Source: CAD feature listing. Evaluate the final solid. Frame: model axes, mm. A direction names the side the tool comes from. Round coordinates to 2 decimals unless told otherwise and drop trailing zeros. Order: outer loops, then holes, each group sorted by start corner. A loop starts at its lowest first (then second) coordinate and runs counter-clockwise, first axis right, second up. Notation, with made-up numbers: (22.5, 86.25) - (64.5, 86.25) arc R36 ccw to (64.5, 120.25) - close; hole circle Ø7 at (-31.75, 73.5). An arc over 180 degrees is marked (long way). Use one line per item in the form item = value. Start each with the question number.
Q1. Ray query, line 1 (X direction, y = 0.5, z = 4.4); line 2 (Y direction, x = 1.5, z = 3.35); line 3 (X direction, y = -2.75, z = 3.8). Return the intervals inside material, ascending. Write a range as [from, to].
Q2. Cut plane C-C, the plane z = 2.85. Give the number of separate pieces and of enclosed holes in the cut face, and give its area (3 significant figures).
Q3. Cut plane A-A, the plane x = -10. Return the cut outline in (y, z), and give its area (3 significant figures).
Q4. Cut plane B-B, the plane y = 0. Return the cut outline in (x, z), and give its area (3 significant figures).
Q5. Draft query along Y for faces 1 (the cylindrical face through (1.576, -5.824, 1.535)), 2 (the cylindrical face through (-14.735, 8.091, 2.958)), 3 (the cylindrical face through (1.576, -5.081, 3.595)), 4 (the flat face through (-5, 3, 0)). Return one class per face: released by +Y, released by -Y, zero draft, split by the parting line, or undercut.
Q6. Set-up query: faces 5 (the flat face through (-5.433, 9, 3)), 6 (the flat face through (-5.704, -3.6, 3)), 7 (the flat face through (-12.199, -3.6, 3)), 8 (the flat face through (-6, 9, 1)). Return all of +Z, -Z, +X, -X, +Y, -Y with unobstructed straight access to the full face (end or side cutting, diameter ignored); none if empty.
Q7. Pin query (flat end, axial travel): pin 1 Ø3 at (x, y) = (-5, 10.5) entering from +Z; pin 2 Ø3 at (y, z) = (-3.5, 3) entering from +X; pin 3 Ø3 at (x, z) = (-11, 3.5) entering from +Y. Return the tip coordinate at first contact, or that it passes through.
Q8. Cut plane D-D, the plane x = 3. Return the cut outline in (y, z).
from build123d import *

# Parameters (mm, degrees)
BOSS_EXTRUDE1_DEPTH            = 4
BOSS_EXTRUDE2_DEPTH            = 1
CUT_EXTRUDE1_DEPTH             = 1
SKETCH4_W                      = 8.3
SKETCH4_H                      = 5
BOSS_EXTRUDE3_DEPTH            = 10
SKETCH5_W                      = 4
SKETCH5_H                      = 0.3
BOSS_EXTRUDE4_DEPTH            = 17.182840277
SKETCH6_W                      = 5
SKETCH6_H                      = 10
BOSS_EXTRUDE5_DEPTH            = 9
SKETCH7_W                      = 5
SKETCH7_H                      = 11
BOSS_EXTRUDE6_DEPTH            = 2.7
BOSS_EXTRUDE7_DEPTH            = 1
SKETCH9_W                      = 2
SKETCH9_H                      = 4
BOSS_EXTRUDE8_DEPTH            = 1.58656304
SKETCH10_W                     = 0.5
SKETCH10_H                     = 3.5
BOSS_EXTRUDE9_DEPTH            = 3.5
SKETCH11_W                     = 0.5
SKETCH11_H                     = 3.5
BOSS_EXTRUDE10_DEPTH           = 3.5
SKETCH12_W                     = 0.5
SKETCH12_H                     = 3.5
BOSS_EXTRUDE11_DEPTH           = 3.5
F_2_5_2_5_DIAMETER_HOLE1_D     = 2.5
F_2_5_2_5_DIAMETER_HOLE1_DEPTH = 6
F_1_5_1_5_DIAMETER_HOLE1_D     = 1.5
F_1_5_1_5_DIAMETER_HOLE1_DEPTH = 3.337462294
F_1_5_1_5_DIAMETER_HOLE2_D     = 1.5
F_1_5_1_5_DIAMETER_HOLE2_DEPTH = 3.641193774
F_1_5_1_5_DIAMETER_HOLE3_D     = 1.5
F_1_5_1_5_DIAMETER_HOLE3_DEPTH = 10.667359759
FILLET1_R                      = 0.5
FILLET2_R                      = 1


with BuildPart() as part:
    # Sketch1 → Boss-Extrude1 (new body)
    with BuildSketch(Plane(origin=(0, 0, 1), x_dir=(-1, 0, 0), z_dir=(0, 0, -1))):
        with BuildLine():
            Line((4.743251359, 8.08281548), (4.036144578, 7.375708699))
            Line((4.036144578, 7.375708699), (12.336144578, 7.375708699))
            Line((12.336144578, 7.375708699), (12.336144578, 9.634817645))
            Line((12.336144578, 9.634817645), (12.079792775, 9.67251644))
            Line((12.079792775, 9.67251644), (12.036144578, 9.375708699))
            Line((12.036144578, 9.375708699), (12.036144578, 8.375708699))
            Line((12.036144578, 8.375708699), (5.450358141, 8.375708699))
            ThreePointArc((5.450358141, 8.375708699), (5.067674708, 8.299588231), (4.743251359, 8.08281548))
        make_face()
    extrude(amount=-BOSS_EXTRUDE1_DEPTH)

    # Sketch2 → Boss-Extrude2 (add)
    with BuildSketch(Plane.XY.offset(5)):
        with BuildLine():
            Line((-12.336144578, 7.375708699), (-12.336144578, 9.634817645))
            Line((-12.336144578, 9.634817645), (-12.079792775, 9.67251644))
            Line((-12.079792775, 9.67251644), (-12.036144578, 9.375708699))
            Line((-12.036144578, 9.375708699), (-12.036144578, 8.375708699))
            Line((-12.036144578, 8.375708699), (-5.450358141, 8.375708699))
            ThreePointArc((-5.450358141, 8.375708699), (-5.067674708, 8.299588231), (-4.743251359, 8.08281548))
            Line((-4.743251359, 8.08281548), (-4.036144578, 7.375708699))
            Line((-4.036144578, 7.375708699), (-12.336144578, 7.375708699))
        make_face()
    extrude(amount=BOSS_EXTRUDE2_DEPTH)

    # Sketch3 → Cut-Extrude1 (cut)
    with BuildSketch(Plane.XY.offset(6)):
        Polygon((-12.036144578, 8.375708699), (-12.036144578, 9.375708699), (-12.079792775, 9.67251644), (-12.336144578, 9.634817645), (-12.336144578, 8.375708699), align=None)
    extrude(amount=-CUT_EXTRUDE1_DEPTH, mode=Mode.SUBTRACT)

    # Sketch4 → Boss-Extrude3 (add)
    with BuildSketch(Plane.XZ.offset(-7.375708699)):
        with Locations((-8.186144578, 3.5)):
            Rectangle(SKETCH4_W, SKETCH4_H)
    extrude(amount=BOSS_EXTRUDE3_DEPTH)

    # Sketch5 → Boss-Extrude4 (add)
    with BuildSketch(Plane(origin=(-10.431763466, -1.534082863, 0), x_dir=(0, 0, -1), z_dir=(0.989359135, 0.14549399, 0))):
        with Locations((-3, 11.177129757)):
            Rectangle(SKETCH5_W, SKETCH5_H)
    extrude(amount=BOSS_EXTRUDE4_DEPTH)

    # Sketch6 → Boss-Extrude5 (add)
    with BuildSketch(Plane(origin=(-4.036144578, 0, 0), x_dir=(0, 0, -1), z_dir=(1, 0, 0))):
        with Locations((-3.5, 2.375708699)):
            Rectangle(SKETCH6_W, SKETCH6_H)
    extrude(amount=BOSS_EXTRUDE5_DEPTH)

    # Sketch7 → Boss-Extrude6 (add)
    with BuildSketch(Plane.ZY.offset(12.336144578)):
        with Locations((3.5, 2.875708699)):
            Rectangle(SKETCH7_W, SKETCH7_H)
    extrude(amount=BOSS_EXTRUDE6_DEPTH)

    # Sketch8 → Boss-Extrude7 (add)
    with BuildSketch(Plane(origin=(0, 0, 1), x_dir=(-1, 0, 0), z_dir=(0, 0, -1))):
        with BuildLine():
            Line((15.036144578, 8.375708699), (15.036144578, -2.624291301))
            Line((15.036144578, -2.624291301), (-4.963855422, -2.624291301))
            Line((-4.963855422, -2.624291301), (-4.963855422, 7.375708699))
            Line((-4.963855422, 7.375708699), (4.036144578, 7.375708699))
            Line((4.036144578, 7.375708699), (4.743251359, 8.08281548))
            ThreePointArc((4.743251359, 8.08281548), (5.067674708, 8.299588231), (5.450358141, 8.375708699))
            Line((5.450358141, 8.375708699), (15.036144578, 8.375708699))
        make_face()
    extrude(amount=BOSS_EXTRUDE7_DEPTH)

    # Sketch9 → Boss-Extrude8 (add)
    with BuildSketch(Plane(origin=(0, 8.375708699, 0), x_dir=(-1, 0, 0), z_dir=(0, 1, 0))):
        with Locations((6.43261709, 3)):
            Rectangle(SKETCH9_W, SKETCH9_H)
    extrude(amount=BOSS_EXTRUDE8_DEPTH)

    # Sketch10 → Boss-Extrude9 (add)
    with BuildSketch(Plane.XZ.offset(2.624291301)):
        with Locations((-5.453504337, 3)):
            Rectangle(SKETCH10_W, SKETCH10_H)
    extrude(amount=BOSS_EXTRUDE9_DEPTH)

    # Sketch11 → Boss-Extrude10 (add)
    with BuildSketch(Plane.XZ.offset(2.624291301)):
        with Locations((1.572661648, 3)):
            Rectangle(SKETCH11_W, SKETCH11_H)
    extrude(amount=BOSS_EXTRUDE10_DEPTH)

    # Sketch12 → Boss-Extrude11 (add)
    with BuildSketch(Plane.XZ.offset(2.624291301)):
        with Locations((-11.948682285, 3)):
            Rectangle(SKETCH12_W, SKETCH12_H)
    extrude(amount=BOSS_EXTRUDE11_DEPTH)

    # Ø2.5 (2.5) Diameter Hole1
    with Locations(Plane.XY.offset(6)):
        with Locations((-9.786144578, 0.375708699), (-0.286144578, 0.375708699)):
            Hole(F_2_5_2_5_DIAMETER_HOLE1_D / 2, depth=F_2_5_2_5_DIAMETER_HOLE1_DEPTH)

    # Ø1.5 (1.5) Diameter Hole1
    with Locations(Plane(origin=(-11.698682285, 0, 0), x_dir=(0, 0, -1), z_dir=(1, 0, 0))):
        with Locations((-3, -4.624291301)):
            Hole(F_1_5_1_5_DIAMETER_HOLE1_D / 2, depth=F_1_5_1_5_DIAMETER_HOLE1_DEPTH)

    # Ø1.5 (1.5) Diameter Hole2
    with Locations(Plane.ZY.offset(-1.322661648)):
        with Locations((3, -4.624291301)):
            Hole(F_1_5_1_5_DIAMETER_HOLE2_D / 2, depth=F_1_5_1_5_DIAMETER_HOLE2_DEPTH)

    # Ø1.5 (1.5) Diameter Hole3
    with Locations(Plane.ZY.offset(5.703504337)):
        with Locations((3, -4.624291301)):
            Hole(F_1_5_1_5_DIAMETER_HOLE3_D / 2, depth=F_1_5_1_5_DIAMETER_HOLE3_DEPTH)

    # Fillet1
    fillet1_edges = [part.edges().sort_by_distance(p)[0] for p in [
        (-7.43261709, 9.962271739, 3),
        (-5.43261709, 9.962271739, 3),
        (-12.336144578, 9.634817645, 3),
        (-12.036144578, 9.375708699, 3),
    ]]
    fillet(fillet1_edges, radius=FILLET1_R)

    # Fillet2
    fillet2_edges = [part.edges().sort_by_distance(p)[0] for p in [
        (-15.036144578, -2.624291301, 3),
        (-15.036144578, 8.375708699, 3),
        (-4.036144578, 7.375708699, 3),
        (-5.453504337, -6.124291301, 1.25),
        (-5.453504337, -6.124291301, 4.75),
        (1.572661648, -6.124291301, 1.25),
        (1.572661648, -6.124291301, 4.75),
        (-11.948682285, -6.124291301, 1.25),
        (-11.948682285, -6.124291301, 4.75),
        (4.963855422, 7.375708699, 3),
        (4.963855422, -2.624291301, 3),
    ]]
    fillet(fillet2_edges, radius=FILLET2_R)


solid = part.part
Completed:
q1.line_1 = [-15.04, -11.03], [-8.54, -1.53], [0.96, 4.96]
q1.line_2 = [-6.12, -5.29], [-3.96, 7.38], [11.37, 11.67]
q1.line_3 = [-12.2, -11.7], [-5.7, -5.2], [1.32, 1.82]
q2.separate_pieces = 4
q2.enclosed_holes = 2
q2.area = 211 mm2
q3.outline = (-2.62, 0) - (-0.86, 0) - (-0.86, 6) - (-2.62, 6) - close; (1.61, 0) - (8.38, 0) - (8.38, 6) - (1.61, 6) - close; (9.68, 1) - (9.98, 1) - (9.98, 5) - (9.68, 5) - close
q3.area = 52.4 mm2
q4.outline = (-15.04, 0) - (-10.98, 0) - (-10.98, 6) - (-15.04, 6) - close; (-8.59, 0) - (-1.48, 0) - (-1.48, 6) - (-8.59, 6) - close; (0.91, 0) - (4.96, 0) - (4.96, 6) - (0.91, 6) - close
q4.area = 91.4 mm2
q5.face_1 = released by -Y
q5.face_2 = released by +Y
q5.face_3 = undercut
q5.face_4 = zero draft
q6.face_5 = +Z, -Z, +X
q6.face_6 = +Z, -Z, -Y
q6.face_7 = +Z, -Z, -X, -Y
q6.face_8 = -Z, +X, -X, +Y
q7.pin_1 = 5
q7.pin_2 = 4.89
q7.pin_3 = 10.05
q8.outline = (-2.62, 0) - (7.38, 0) - (7.38, 6) - (-2.62, 6) - close; (11.59, 1) - (11.89, 1) - (11.89, 5) - (11.59, 5) - close
